Verification items for the finished model (mm, model axes). A direction names the side the tool comes from. Coordinates: 2 decimals unless noted, no trailing zeros. Order: outer loops, then holes, each group sorted by start corner. A loop starts at its lowest first (then second) coordinate and runs counter-clockwise, first axis right, second up. Notation, with made-up numbers: (-36.5, 72) -> (5.5, 72) arc R33 ccw to (5.5, 102) -> close; hole circle Ø1 at (0.5, 86.5). An arc over 180 degrees is marked (long way). Use CSV: the item, a comma, the result in double quotes. Start each with the question number.
1) Release check for a two-part mould opening along Y. For faces 4 (the flat face through (18, -1, 1)), 5 (the cylindrical face through (-1, -0.98, 1.01)), 6 (the flat face through (22, 22, 0)) record: released by +Y, released by -Y, zero draft, split by the parting line, or undercut.
2) Sectioned sample at A-A on x = 36.5. Record the boundary of the cut face in (y, z).
3) Sectioned sample at B-B on z = 0.6. Record the boundary of the cut face in (x, y), then the cut area to 3 significant figures.
4) Scan lines: line 1 along X through (y, z) = (38, 0.55); line 2 along Z through (x, y) = (23.5, 30.5). Record each from-to range of solid material in increasing order.
5) Tool access check on faces 1 (the flat face through (27, -1, 1)), 2 (the cylindrical face through (46, 45.98, 1.01)), 3 (the flat face through (0, 22, 1)). Record the directions out of +Z, -Z, +X, -X, +Y, -Y that give a thin tool (end or side, any length) a straight path to the whole face; none if there is none.
6) Go/stop test with flat-tipped pins: pin 1 (1 mm diameter, centred on x = 39, z = -1, fed in from +Y); pin 2 (0.7 mm diameter, centred on y = -1, z = 1, fed in from +X); pin 3 (22.5 mm diameter, centred on x = 18, y = 32.5, fed in from +Z). Record where each tip stops, or that it passes through.
from build123d import *

# Parameters (mm, degrees)
SKETCH_W     = 45
SKETCH_H     = 45
PAD_DEPTH    = 2
THICKNESS_T  = 1.4
SKETCH001_W  = 9
SKETCH001_H  = 1.4
POCKET_DEPTH = 2


with BuildPart() as part:
    # Sketch → Pad (new body)
    with BuildSketch(Plane.XY):
        with Locations((22.5, 22.5)):
            Rectangle(SKETCH_W, SKETCH_H)
    extrude(amount=PAD_DEPTH)

    # Thickness
    thickness_openings = [part.faces().sort_by_distance(p)[0] for p in [
        (22.5, 22.5, 2),
    ]]
    offset(amount=THICKNESS_T, openings=thickness_openings)

    # Sketch001 → Pocket (cut)
    with BuildSketch(Plane.XY.offset(2)):
        with Locations((22.5, -0.7)):
            Rectangle(SKETCH001_W, SKETCH001_H)
    extrude(amount=-POCKET_DEPTH, mode=Mode.SUBTRACT)


solid = part.part
Answers follow:
1,face 4,"zero draft"
1,face 5,"released by -Y"
1,face 6,"undercut"
2,outline,"(-1.4, 0) arc R1.4 ccw to (0, -1.4) -> (45, -1.4) arc R1.4 ccw to (46.4, 0) -> (46.4, 2) -> (45, 2) -> (45, 0) -> (0, 0) -> (0, 2) -> (-1.4, 2) -> close"
3,outline,"(-1.4, 0) arc R1.4 ccw to (0, -1.4) -> (18, -1.4) -> (18, 0) -> (0, 0) -> (0, 45) -> (45, 45) -> (45, 0) -> (27, 0) -> (27, -1.4) -> (45, -1.4) arc R1.4 ccw to (46.4, 0) -> (46.4, 45) arc R1.4 ccw to (45, 46.4) -> (0, 46.4) arc R1.4 ccw to (-1.4, 45) -> close"
3,area,"246 mm²"
4,line 1,"x = -1.4 to 0, 45 to 46.4"
4,line 2,"z = -1.4 to 0"
5,face 1,"+Z, -Y"
5,face 2,"+Z, -Z, +X, +Y"
5,face 3,"+Z"
6,pin 1,"stops at y = 46.31"
6,pin 2,"stops at x = 46.24"
6,pin 3,"stops at z = 0"
